Geometry: final body of the model. Coordinates: model frame, mm. Face numbers are marked on the shaded views. A direction names the side the tool comes from. Coordinates: 2 decimals unless noted, no trailing zeros. Loops run counter-clockwise (first coordinate to the right, second up) from the corner with the lowest first, then second, coordinate; pieces in that order, holes last. Notation, with made-up numbers: (-10.75, 46.25) -> (18.25, 46.25) arc R22 ccw to (18.25, 78.25) -> close; hole circle Ø6 at (32.5, 58). An arc over 180 degrees is marked (long way). One line per item, written item: value. Start each with the question number.
from build123d import *

# Parameters (mm, degrees)
SKETCH3_W           = 381
SKETCH3_H           = 111.76
BOSS_EXTRUDE1_DEPTH = 34.29
SKETCH2_4_R         = 29.21
CUT_EXTRUDE2_DEPTH  = 127
CUT_EXTRUDE3_START  = 8.89
SKETCH2_5_W         = 119.507
SKETCH2_5_H         = 82.804
CUT_EXTRUDE3_DEPTH  = 127
CUT_EXTRUDE4_START  = 8.89
SKETCH2_W           = 6.604
SKETCH2_H           = 8.636
CUT_EXTRUDE4_DEPTH  = 127
CUT_EXTRUDE6_DEPTH  = 127
CUT_EXTRUDE7_DEPTH  = 127
SKETCH7_W           = 19.689939458
SKETCH7_H           = 8.636
CUT_EXTRUDE8_DEPTH  = 25.4
SKETCH8_W           = 102.108
SKETCH8_H           = 102.108
CUT_EXTRUDE9_DEPTH  = 5.08
SKETCH9_R           = 7.5
CUT_EXTRUDE10_DEPTH = 12.7
SKETCH10_R          = 3.5
CUT_EXTRUDE11_DEPTH = 55.372
CUT_EXTRUDE12_DEPTH = 15.24
SKETCH12_R          = 3.25
SKETCH12_R_2        = 3.5
CUT_EXTRUDE13_DEPTH = 12.446
SKETCH13_R          = 7.5
CUT_EXTRUDE14_DEPTH = 5.08
SKETCH14_W          = 127
SKETCH14_H          = 13.97
SKETCH14_W_2        = 24.003
SKETCH14_H_2        = 39.37
SKETCH14_W_3        = 15.24
SKETCH14_H_3        = 60.96
CUT_EXTRUDE15_DEPTH = 25.4


with BuildPart() as part:
    # Sketch3 → Boss-Extrude1 (new body)
    with BuildSketch(Plane(origin=(0, 0, 0), x_dir=(1, 0, 0), z_dir=(0, 1, 0))):
        with Locations((139.7, 36.195)):
            Rectangle(SKETCH3_W, SKETCH3_H)
    extrude(amount=BOSS_EXTRUDE1_DEPTH)

    # Sketch2<4> → Cut-Extrude2 (cut)
    with BuildSketch(Plane(origin=(0, 0, 0), x_dir=(1, 0, 0), z_dir=(0, 1, 0))):
        with Locations(Location((273.05, 36.195, 0), (0, 0, 270))):
            Circle(SKETCH2_4_R)
    extrude(amount=CUT_EXTRUDE2_DEPTH, mode=Mode.SUBTRACT)

    # Sketch2<5> → Cut-Extrude3 (cut)
    with BuildSketch(Plane(origin=(0, 0, 0), x_dir=(1, 0, 0), z_dir=(0, 1, 0)).offset(CUT_EXTRUDE3_START)):
        with Locations((246.3165, 44.577)):
            Rectangle(SKETCH2_5_W, SKETCH2_5_H)
    extrude(amount=CUT_EXTRUDE3_DEPTH, mode=Mode.SUBTRACT)

    # Sketch2 → Cut-Extrude4 (cut)
    with BuildSketch(Plane(origin=(0, 0, 0), x_dir=(1, 0, 0), z_dir=(0, 1, 0)).offset(CUT_EXTRUDE4_START)):
        Polygon((174.244, 48.895), (186.563, 48.895), (186.563, 77.089), (174.244, 77.089), (174.244, 68.453), align=None)
        with Locations((170.942, 72.771)):
            Rectangle(SKETCH2_W, SKETCH2_H)
    extrude(amount=CUT_EXTRUDE4_DEPTH, mode=Mode.SUBTRACT)

    # Sketch4 → Cut-Extrude6 (cut)
    with BuildSketch(Plane(origin=(0, 34.29, 0), x_dir=(1, 0, 0), z_dir=(0, 1, 0))):
        Polygon((152.4, 48.895), (127, 61.595), (127, 10.795), (152.4, 23.495), (152.4, -19.685), (-50.8, -19.685), (-50.8, 92.075), (152.4, 92.075), align=None)
    extrude(amount=-CUT_EXTRUDE6_DEPTH, mode=Mode.SUBTRACT)

    # Sketch6 → Cut-Extrude7 (cut)
    with BuildSketch(Plane.XY.offset(19.685)):
        Polygon((127, 34.29), (136.187977808, 0), (101.054732315, 0), align=None)
    extrude(amount=-CUT_EXTRUDE7_DEPTH, mode=Mode.SUBTRACT)

    # Sketch7 → Cut-Extrude8 (cut)
    with BuildSketch(Plane(origin=(0, 34.29, 0), x_dir=(1, 0, 0), z_dir=(0, 1, 0))):
        with Locations((157.795030271, 72.771)):
            Rectangle(SKETCH7_W, SKETCH7_H)
    extrude(amount=-CUT_EXTRUDE8_DEPTH, mode=Mode.SUBTRACT)

    # Sketch8 → Cut-Extrude9 (cut)
    with BuildSketch(Plane.XZ):
        with Locations((273.05, -36.195)):
            Rectangle(SKETCH8_W, SKETCH8_H)
    extrude(amount=-CUT_EXTRUDE9_DEPTH, mode=Mode.SUBTRACT)

    # Sketch9 → Cut-Extrude10 (cut)
    with BuildSketch(Plane(origin=(0, 34.29, 0), x_dir=(1, 0, 0), z_dir=(0, 1, 0))):
        with Locations(Location((317.5, 79.375, 0), (0, 0, 270))):
            Circle(SKETCH9_R)
        with Locations(Location((317.5, -6.985, 0), (0, 0, 270))):
            Circle(SKETCH9_R)
        with Locations((165.1, 79.375)):
            Circle(SKETCH9_R)
        with Locations(Location((165.1, -6.985, 0), (0, 0, 270))):
            Circle(SKETCH9_R)
    extrude(amount=-CUT_EXTRUDE10_DEPTH, mode=Mode.SUBTRACT)

    # Sketch10 → Cut-Extrude11 (cut)
    with BuildSketch(Plane(origin=(0, 21.59, 0), x_dir=(1, 0, 0), z_dir=(0, 1, 0))):
        with Locations(Location((317.5, 79.375, 0), (0, 0, 270))):
            Circle(SKETCH10_R)
        with Locations(Location((317.5, -6.985, 0), (0, 0, 270))):
            Circle(SKETCH10_R)
        with Locations(Location((165.1, -6.985, 0), (0, 0, 270))):
            Circle(SKETCH10_R)
        with Locations(Location((165.1, 79.375, 0), (0, 0, 270))):
            Circle(SKETCH10_R)
    extrude(amount=-CUT_EXTRUDE11_DEPTH, mode=Mode.SUBTRACT)

    # Sketch11 → Cut-Extrude12 (cut)
    with BuildSketch(Plane.XZ):
        Polygon((159.6, -82.550426481), (165.1, -85.725852961), (170.6, -82.550426481), (170.6, -76.199573519), (165.1, -73.024147039), (159.6, -76.199573519), align=None)
        Polygon((312, 3.809573519), (317.5, 0.634147039), (323, 3.809573519), (323, 10.160426481), (317.5, 13.335852961), (312, 10.160426481), align=None)
        Polygon((165.1, 0.634147039), (170.6, 3.809573519), (170.6, 10.160426481), (165.1, 13.335852961), (159.6, 10.160426481), (159.6, 3.809573519), align=None)
        Polygon((317.5, -85.725852961), (323, -82.550426481), (323, -76.199573519), (317.5, -73.024147039), (312, -76.199573519), (312, -82.550426481), align=None)
    extrude(amount=-CUT_EXTRUDE12_DEPTH, mode=Mode.SUBTRACT)

    # Sketch12 → Cut-Extrude13 (cut)
    with BuildSketch(Plane(origin=(0, 8.89, 0), x_dir=(1, 0, 0), z_dir=(0, 1, 0))):
        with Locations(Location((230.55, 34.395, 0), (0, 0, 270))):
            Circle(SKETCH12_R)
        with Locations(Location((218.05, 46.895, 0), (0, 0, 270))):
            Circle(SKETCH12_R_2)
    extrude(amount=-CUT_EXTRUDE13_DEPTH, mode=Mode.SUBTRACT)

    # Sketch13 → Cut-Extrude14 (cut)
    with BuildSketch(Plane.XZ):
        with Locations((218.05, -46.895)):
            Circle(SKETCH13_R)
    extrude(amount=-CUT_EXTRUDE14_DEPTH, mode=Mode.SUBTRACT)

    # Sketch14 → Cut-Extrude15 (cut)
    with BuildSketch(Plane(origin=(0, 34.29, 0), x_dir=(1, 0, 0), z_dir=(0, 1, 0))):
        with Locations((241.3, -7.62)):
            Rectangle(SKETCH14_W, SKETCH14_H)
        with Locations((170.7515, 25.4)):
            Rectangle(SKETCH14_W_2, SKETCH14_H_2)
        with Locations((317.5, 36.195)):
            Rectangle(SKETCH14_W_3, SKETCH14_H_3)
    extrude(amount=-CUT_EXTRUDE15_DEPTH, mode=Mode.SUBTRACT)


solid = part.part
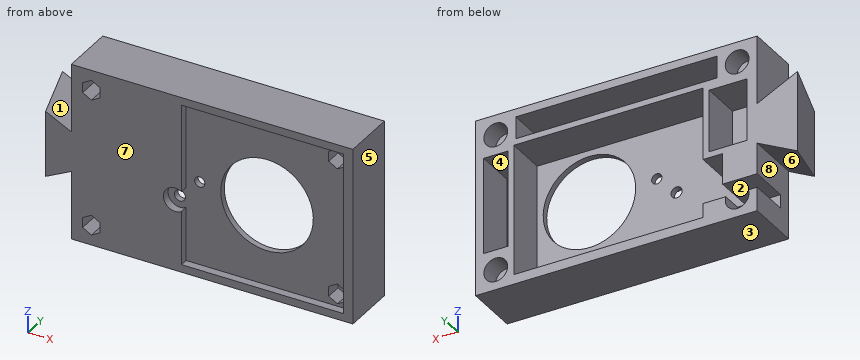
1. Section A-A on x = 218.05. Return the cut outline in (y, z) (3 decimals), plus the area to 3 significant figures.
2. Section D-D on y = 24. Count the separate pieces of the cut face and the enclosed holes in it, plus the area to 3 significant figures.
3. Section B-B on x = 194. Return the cut outline in (y, z) (3 decimals).
4. Pin query (flat end, axial travel): pin 1 Ø3 at (y, z) = (16.5, -53) entering from -X; pin 2 Ø12 at (y, z) = (4, -74.5) entering from -X; pin 3 Ø1.5 at (x, z) = (278, -63) entering from -Y; pin 4 Ø12 at (x, z) = (317.5, 8) entering from -Y. Return the tip coordinate at first contact, or that it passes through.
5. Section C-C on x = 273.05. Return the cut outline in (y, z) (3 decimals).
6. Line query: L1, parallel to Z at x = 317.5, y = 19.25 (3 decimals); L2, parallel to X at y = 16, z = -9.5; L3, parallel to Z at x = 263.5, y = 30 (3 decimals). Output: solid intervals per line, ascending. Write a range as [from, to].
7. Set-up query: the marked faces 1, 2, 3 and 4. Return all of +Z, -Z, +X, -X, +Y, -Y with unobstructed straight access to the full face (end or side cutting, diameter ignored); none if empty.
8. Draft query along X for the marked faces 5, 6, 7 and 8. Return one class per face: released by +X, released by -X, zero draft, split by the parting line, or undercut.
Checks:
1. outline: (0, -92.075) -> (34.29, -92.075) -> (34.29, -85.979) -> (8.89, -85.979) -> (8.89, -50.395) -> (5.08, -50.395) -> (5.08, -54.395) -> (0, -54.395) -> close; (0, -39.395) -> (5.08, -39.395) -> (5.08, -43.395) -> (8.89, -43.395) -> (8.89, -3.175) -> (34.29, -3.175) -> (34.29, 0.635) -> (8.89, 0.635) -> (8.89, 14.605) -> (34.29, 14.605) -> (34.29, 19.685) -> (0, 19.685) -> close
1. area: 1,270 mm²
2. separate pieces: 1
2. enclosed holes: 6
2. area: 5,970 mm²
3. outline: (0, -92.075) -> (34.29, -92.075) -> (34.29, -85.979) -> (8.89, -85.979) -> (8.89, -3.175) -> (34.29, -3.175) -> (34.29, 0.635) -> (8.89, 0.635) -> (8.89, 14.605) -> (34.29, 14.605) -> (34.29, 19.685) -> (0, 19.685) -> close
4. pin 1: x = 131.36
4. pin 2: x = 152.4
4. pin 3: through
4. pin 4: y = 5.08
5. outline: (0, -92.075) -> (34.29, -92.075) -> (34.29, -85.979) -> (8.89, -85.979) -> (8.89, -65.405) -> (5.08, -65.405) -> (5.08, -87.249) -> (0, -87.249) -> close; (0, 14.859) -> (5.08, 14.859) -> (5.08, -6.985) -> (8.89, -6.985) -> (8.89, -3.175) -> (34.29, -3.175) -> (34.29, 0.635) -> (8.89, 0.635) -> (8.89, 14.605) -> (34.29, 14.605) -> (34.29, 19.685) -> (0, 19.685) -> close
6. L1: [-92.075, -82.875], [-75.875, -66.675], [-5.715, 3.485], [10.485, 19.685]
6. L2: [152.4, 158.75], [182.75, 186.56], [306.07, 309.88], [325.12, 330.2]
6. L3: [-92.075, -85.979], [-3.175, 0.635], [14.605, 19.685]
7. face 1: +Z, +Y, -Y
7. face 2: -X, +Y
7. face 3: -Z, +X, -X, +Y, -Y
7. face 4: +Y
8. face 5: released by +X
8. face 6: undercut
8. face 7: zero draft
8. face 8: undercut
